from build123d import *

# Parameters (mm, degrees)
SKETCH1_W               = 48
SKETCH1_H               = 26
BOSS_EXTRUDE1_DEPTH     = 8
CUT_EXTRUDE1_DEPTH      = 1
CUT_EXTRUDE1_DEPTH_BACK = 49
FILLET1_R               = 2
SKETCH5_W               = 26
SKETCH5_H               = 2
BOSS_EXTRUDE2_DEPTH     = 10
SKETCH6_R               = 1.5
CUT_EXTRUDE2_DEPTH      = 10
SKETCH3_W               = 10
SKETCH3_H               = 2
CUT_EXTRUDE3_DEPTH      = 27
FILLET3_R               = 2
SKETCH7_R               = 4
SKETCH7_R_2             = 1.5
BOSS_EXTRUDE3_DEPTH     = 2


with BuildPart() as part:
    # Sketch1 → Boss-Extrude1 (new body)
    with BuildSketch(Plane(origin=(0, 0, 0), x_dir=(1, 0, 0), z_dir=(0, 1, 0))):
        Rectangle(SKETCH1_W, SKETCH1_H)
    extrude(amount=-BOSS_EXTRUDE1_DEPTH)

    # Sketch2 → Cut-Extrude1 (cut, two sides)
    with BuildSketch(Plane(origin=(24, 0, 0), x_dir=(0, 0, -1), z_dir=(1, 0, 0))) as cut_extrude1_sk:
        Polygon((-8, -5), (-13, -8), (0, -8), (0, -5), align=None)
        Polygon((0, -5), (0, -8), (13, -8), (8, -5), align=None)
    extrude(amount=CUT_EXTRUDE1_DEPTH, mode=Mode.SUBTRACT)
    extrude(cut_extrude1_sk.sketch, amount=-CUT_EXTRUDE1_DEPTH_BACK, mode=Mode.SUBTRACT)

    # Fillet1
    fillet1_edges = [part.edges().sort_by_distance(p)[0] for p in [
        (0, -8, -13),
        (0, -5, 8),
        (0, -5, -8),
        (0, -8, 13),
    ]]
    fillet(fillet1_edges, radius=FILLET1_R)

    # Sketch5 → Boss-Extrude2 (add)
    with BuildSketch(Plane.ZY.offset(24)):
        with Locations((0, -1)):
            Rectangle(SKETCH5_W, SKETCH5_H)
    boss_extrude2 = extrude(amount=BOSS_EXTRUDE2_DEPTH)

    # Mirror1: Boss-Extrude2 across plane
    add(boss_extrude2.mirror(Plane(origin=(0, 0, 0), x_dir=(0, 0, 1), z_dir=(1, 0, 0))))

    # Sketch6 → Cut-Extrude2 (cut)
    with BuildSketch(Plane(origin=(0, 0, 0), x_dir=(1, 0, 0), z_dir=(0, 1, 0))):
        with Locations((-30, 11)):
            Circle(SKETCH6_R)
        with Locations((-30, -11)):
            Circle(SKETCH6_R)
        with Locations((30, -11)):
            Circle(SKETCH6_R)
        with Locations((30, 11)):
            Circle(SKETCH6_R)
    extrude(amount=-CUT_EXTRUDE2_DEPTH, mode=Mode.SUBTRACT)

    # Sketch3 → Cut-Extrude3 (cut, through all)
    with BuildSketch(Plane.XY.offset(13)):
        with Locations((5, -1)):
            Rectangle(SKETCH3_W, SKETCH3_H)
        with Locations((-5, -1)):
            Rectangle(SKETCH3_W, SKETCH3_H)
    extrude(amount=-CUT_EXTRUDE3_DEPTH, mode=Mode.SUBTRACT)

    # Fillet3
    fillet3_edges = [part.edges().sort_by_distance(p)[0] for p in [
        (-34, -1, -13),
        (-34, -1, 13),
        (34, -1, -13),
        (34, -1, 13),
    ]]
    fillet(fillet3_edges, radius=FILLET3_R)

    # Sketch7 → Boss-Extrude3 (add)
    with BuildSketch(Plane(origin=(0, 0, 0), x_dir=(1, 0, 0), z_dir=(0, 1, 0))):
        with BuildLine():
            Line((-32, 13), (-26.535898385, 13))
            ThreePointArc((-26.535898385, 13), (-31.03527618, 14.863703305), (-34, 11))
            ThreePointArc((-34, 11), (-33.414213562, 12.414213562), (-32, 13))
        make_face()
        with BuildLine():
            ThreePointArc((-34, -11), (-31.03527618, -14.863703305), (-26.535898385, -13))
            Line((-26.535898385, -13), (-32, -13))
            ThreePointArc((-32, -13), (-33.414213562, -12.414213562), (-34, -11))
        make_face()
        with Locations((30, 11)):
            Circle(SKETCH7_R)
        with Locations((30, 11)):
            Circle(SKETCH7_R_2, mode=Mode.SUBTRACT)
        with Locations((30, -11)):
            Circle(SKETCH7_R)
        with Locations((30, -11)):
            Circle(SKETCH7_R_2, mode=Mode.SUBTRACT)
    extrude(amount=-BOSS_EXTRUDE3_DEPTH)


solid = part.part
Design review of the part built by this model. Coordinates are the model's own, in mm. A direction names the side the tool comes from. Give positions to 0.01 mm unless a question says otherwise; leave off trailing zeros. Loops run counter-clockwise (first coordinate to the right, second up) from the corner with the lowest first, then second, coordinate; pieces in that order, holes last. Notation, with made-up numbers: (26, -17.75) -> (59, -17.75) arc R27 ccw to (59, 10.25) -> close; hole circle Ø6 at (81.25, 1). An arc over 180 degrees is marked (long way). One line per question, with ' | ' between items. Start each with the question number.
(1) Draft analysis for pull direction Z (two halves, no side actions). For faces 4 (the face through (-22, 0, 0)), 5 (the face through (-0.4, -2.3, 13)), 6 (the face through (0.3, -6.2, -12)), state which applies: +Z half, -Z half, draft (parallel to the pull), parting line (faces both ways), or undercut.
(2) Insertion check: P1, Ø2.5, axis at x = -30, z = -11, coming from the -Y side; P2, Ø3, axis at x = 30.5, z = 0, coming from the -Y side; P3, Ø4.5, axis at x = -8.5, z = -1, coming from the -Y side; P4, Ø2, axis at x = -8.5, y = -1.5, coming from the -Z side. Each pin has a flat end and moves straight along its axis. Give the tip position at first contact, or say it passes through.
(3) We need section D-D (y = -3.5). State the section outline as (x, z) points.
(4) We need section C-C (x = 2.5). State the section outline as (y, z) points, and give its area (3 significant figures).
(5) For line 1 (X direction, y = -1.6, z = 11); line 2 (Z direction, x = -30, y = -1); line 3 (X direction, y = -1.5, z = -4), list the stretches that pass through material, from the lowest coordinate up.
(6) For faces 1 (the face through (0, -5, 0)), 2 (the face through (-29, -2, 0)), 3 (the face through (-0.4, -2.3, -13)), list the 3-axis set-ups (+Z, -Z, +X, -X, +Y, -Y) from which the entire face can be reached by the end or side of a thin tool; tool diameter is ignored.
(7) We need section A-A (x = -30). State the section outline as (y, z) points.
(8) We need section B-B (z = 6.75). State the section outline as (x, y) points, and give its area (3 significant figures).
The answers:
1) face 4: draft | face 5: +Z half | face 6: undercut
2) P1: passes through | P2: stops at y = -2 | P3: stops at y = -5 | P4: stops at z = -13
3) outline: (-24, -13) -> (24, -13) -> (24, 13) -> (-24, 13) -> close
4) outline: (-6.18, -9.97) arc R2 ccw to (-4.47, -13) -> (-2, -13) -> (-2, 13) -> (-4.47, 13) arc R2 ccw to (-6.18, 9.97) -> (-5.29, 8.48) arc R2 cw to (-5, 7.45) -> (-5, -7.45) arc R2 cw to (-5.29, -8.48) -> close | area: 87.4 mm^2
5) line 1: x = -34 to -31.5, -28.5 to -10, 10 to 28.5, 31.5 to 34 | line 2: z = -15 to -12.5, -9.5 to 9.5, 12.5 to 15 | line 3: x = -34 to -10, 10 to 34
6) face 1: +X, -X, -Y | face 2: +Z, -Z, -X, -Y | face 3: -Z, +Y, -Y
7) outline: (-2, -15) -> (0, -15) -> (0, -12.5) -> (-2, -12.5) -> close; (-2, -9.5) -> (0, -9.5) -> (0, 9.5) -> (-2, 9.5) -> close; (-2, 12.5) -> (0, 12.5) -> (0, 15) -> (-2, 15) -> close
8) outline: (-34, -2) -> (-24, -2) -> (-24, -5) -> (24, -5) -> (24, -2) -> (34, -2) -> (34, 0) -> (10, 0) -> (10, -2) -> (-10, -2) -> (-10, 0) -> (-34, 0) -> close | area: 240 mm^2
